Part model, mm, in its own coordinate system. Face numbers are marked on the shaded views. Give positions to 0.01 mm unless a question says otherwise; leave off trailing zeros. Order: outer loops, then holes, each group sorted by start corner. A loop starts at its lowest first (then second) coordinate and runs counter-clockwise, first axis right, second up. Notation, with made-up numbers: (-29, 48) - (8, 48) arc R21 cw to (8, 58) - close; hole circle Ø6 at (50.5, 71). An arc over 180 degrees is marked (long way). One line per item, written item: value.
```python
from build123d import *

# Parameters (mm, degrees)
SKETCH_1_W          = 98
SKETCH_1_H          = 20
EXTRUDE_1_DEPTH     = 7
EXTRUDE_2_DEPTH     = 98
CUT_EXTRUDE_START   = -6
SKETCH_3_R          = 2.5
SKETCH_3_R_2        = 1.5
CUT_EXTRUDE_3_DEPTH = 98
SKETCH_4_R          = 1.5
CUT_EXTRUDE_6_DEPTH = 98


with BuildPart() as part:
    # 草图1 → 凸台-拉伸1 (new body)
    with BuildSketch(Plane.XY):
        with Locations((0.769633508, 15.397905759)):
            Rectangle(SKETCH_1_W, SKETCH_1_H)
    extrude(amount=EXTRUDE_1_DEPTH)

    # 草图2 → 凸台-拉伸2 (add)
    with BuildSketch(Plane.ZY.offset(48.230366492)):
        Polygon((7, 25.397905759), (7, 5.397905759), (12.864294632, 5.397905759), (16.347940075, 5.397905759), align=None)
    extrude(amount=-EXTRUDE_2_DEPTH)

    # 草图3 → 切除-拉伸3 (cut)
    # profile 1 of 2: a face of its own
    with BuildSketch(Plane(origin=(0, 0, 0), x_dir=(-1, 0, 0), z_dir=(0, 0, -1)).offset(CUT_EXTRUDE_START)):
        with Locations((-44.769633508, 15.397905759)):
            Circle(SKETCH_3_R)
    # profile 2 of 2: a face of its own
    with BuildSketch(Plane(origin=(0, 0, 0), x_dir=(-1, 0, 0), z_dir=(0, 0, -1)).offset(CUT_EXTRUDE_START)):
        with Locations((43.230366492, 15.397905759)):
            Circle(SKETCH_3_R)
        with Locations((43.230366492, 15.397905759)):
            Circle(SKETCH_3_R_2, mode=Mode.SUBTRACT)
    extrude(amount=-CUT_EXTRUDE_3_DEPTH, mode=Mode.SUBTRACT)

    # 草图4 → 切除-拉伸6 (cut)
    with BuildSketch(Plane.XY):
        with Locations(Location((-43.230366492, 15.397905759, 0), (0, 0, 180))):
            Circle(SKETCH_4_R)
        with Locations(Location((44.769633508, 15.397905759, 0), (0, 0, 180))):
            Circle(SKETCH_4_R)
    extrude(amount=CUT_EXTRUDE_6_DEPTH, mode=Mode.SUBTRACT)


solid = part.part
```
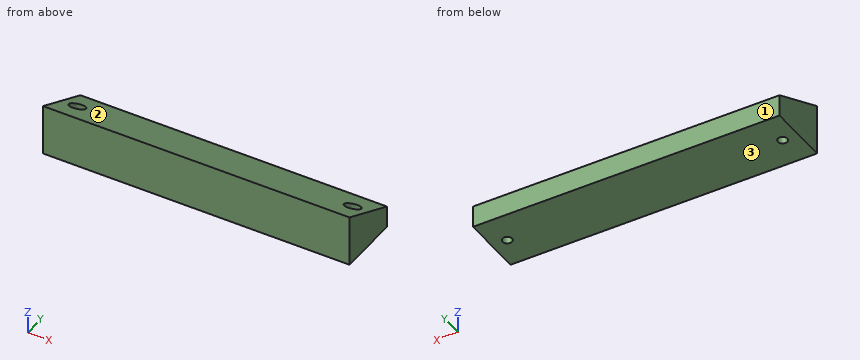
1) Slice it at B-B on x = -9. Write the cut outline in (y, z), then the cut area to 3 significant figures.
Answer:
outline: (5.4, 0) - (25.4, 0) - (25.4, 7) - (5.4, 16.35) - close
area: 233 mm2
2) Slice it at C-C on y = 21.75. Write the cut outline in (x, z).
Answer:
outline: (-48.23, 0) - (49.77, 0) - (49.77, 8.71) - (-48.23, 8.71) - close
3) Drop flat-ended pins along their axis: P1, Ø5.5, axis at x = -42.5, y = 14.5, coming from the +Z side; P2, Ø5.5, axis at x = 45.5, y = 16, coming from the +Z side; P3, Ø1.5, axis at x = -25, y = 18, coming from the +Z side. Give the stop position or say it passes through.
Answer:
P1: stops at z = 13.38
P2: stops at z = 12.64
P3: stops at z = 10.81
4) Two-plate mould, pull along Z, no slides. Class the marked faces 1, 2 and 3: pulls with the +Z half, pulls with the -Z half, needs draft (parallel to the pull), parting line crosses it, or undercut.
Answer:
face 1: needs draft
face 2: pulls with the +Z half
face 3: pulls with the -Z half
5) Slice it at A-A on z = 10.5. Write the cut outline in (x, y), then the cut area to 3 significant figures.
Answer:
outline: (-48.23, 5.4) - (49.77, 5.4) - (49.77, 17.91) - (-48.23, 17.91) - close; hole circle Ø5 at (-43.23, 15.4); hole circle Ø5 at (44.77, 15.4)
area: 1,190 mm2
6) Wall check: line 1 along Y through (x, z) = (42.5, 9); line 2 along Z through (x, y) = (23.5, 13.5); line 3 along Y through (x, z) = (-5.5, 15). Give the ranges that are in metal, low to high. Write a range as [from, to].
Answer:
line 1: y = [5.4, 14.35], [16.45, 21.12]
line 2: z = [0, 12.56]
line 3: y = [5.4, 8.28]
